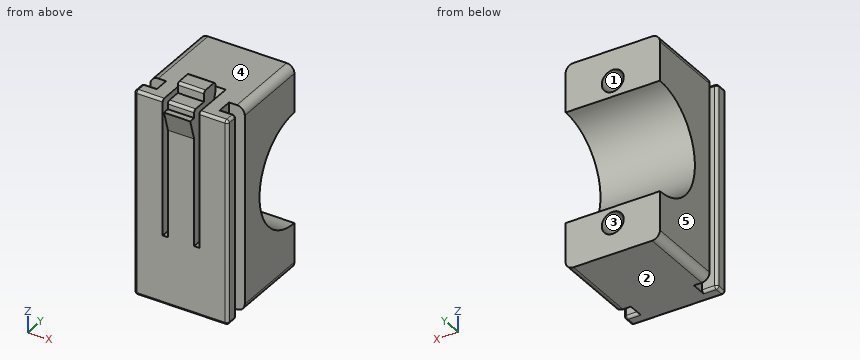
from build123d import *

# Parameters (mm, degrees)
BOSS_EXTRUDE1_DEPTH             = 39
HANDLEBARHOLE_R                 = 10.55
CUT_EXTRUDE1_DEPTH              = 48.381430962
SKETCH3_R                       = 2.1
CUT_EXTRUDE2_DEPTH              = 14
BOSS_EXTRUDE2_DEPTH             = 2.5
BOSS_EXTRUDE2_DEPTH_BACK        = 2.5
FILLET1_R                       = 0.5
CUT_EXTRUDE_THIN2_START         = -3.5
CUT_EXTRUDE_THIN2_DEPTH         = 7
CUT_EXTRUDE5_REACH              = 49.381
SKETCH10_W                      = 1
SKETCH10_H                      = 25.953669743
BOSS_EXTRUDE3_REACH             = 46.744
BOSS_EXTRUDE3_DIRECTION_2_REACH = 46.744
FILLET5_R                       = 1.5


# Read off the part's stored shape, not the designer's step: Cut-Extrude-Thin2
with BuildPart() as part:
    # Sketch1 → Boss-Extrude1 (new body)
    with BuildSketch(Plane.XY):
        Polygon((0, 5), (0, 20), (18, 20), (18, 5), (15, 5), (15, 2.5), (17.9, 2.5), (17.9, 0), (0.1, 0), (0.1, 2.5), (3, 2.5), (3, 5), align=None)
    extrude(amount=BOSS_EXTRUDE1_DEPTH)

    # HandlebarHole → Cut-Extrude1 (cut, through all)
    with BuildSketch(Plane(origin=(0, 0, 0), x_dir=(0, 0, -1), z_dir=(1, 0, 0))):
        with Locations((-19.5, 20)):
            Circle(HANDLEBARHOLE_R)
    extrude(amount=CUT_EXTRUDE1_DEPTH, mode=Mode.SUBTRACT)

    # Sketch3 → Cut-Extrude2 (cut)
    with BuildSketch(Plane(origin=(0, 20, 0), x_dir=(1, 0, 0), z_dir=(0, 1, 0))):
        with Locations(Location((9, -5.95, 0), (0, 0, 270))):
            Circle(SKETCH3_R)
        with Locations(Location((9, -33.05, 0), (0, 0, 270))):
            Circle(SKETCH3_R)
    extrude(amount=-CUT_EXTRUDE2_DEPTH, mode=Mode.SUBTRACT)

    # Sketch4 → Boss-Extrude2 (add, two sides: drawn at the far end of the back side and taken through both)
    with BuildSketch(Plane.ZY.offset(-9).offset(-BOSS_EXTRUDE2_DEPTH_BACK)):
        Polygon((33.5, 0), (37.5, 0), (37.5, -1.2), align=None)
    extrude(amount=BOSS_EXTRUDE2_DEPTH + BOSS_EXTRUDE2_DEPTH_BACK)

    # Fillet1
    fillet1_edges = [part.edges().sort_by_distance(p)[0] for p in [
        (17.9, 1.25, 39),
        (1.55, 2.5, 0),
        (16.45, 2.5, 39),
        (16.45, 2.5, 0),
        (17.9, 1.25, 0),
        (9, 0, 0),
        (0.1, 1.25, 0),
        (0.1, 2.5, 19.5),
        (17.9, 2.5, 19.5),
        (17.9, 0, 19.5),
        (0.1, 0, 19.5),
        (1.55, 2.5, 39),
        (0.1, 1.25, 39),
        (9, 0, 39),
    ]]
    fillet(fillet1_edges, radius=FILLET1_R)

    # Cut-Extrude-Thin2 outline → Cut-Extrude-Thin2 (cut)
    with BuildSketch(Plane.ZY.offset(-9).offset(CUT_EXTRUDE_THIN2_START)):
        with BuildLine():
            add(Edge.make_bspline(
                [(39, 6.377827527), (26.271218228, 2.589898365), (13, 3)],
                knots=[0.07295309, 0.07295309, 0.07295309, 1, 1, 1], degree=2))
            Line((39, 6.377827527), (39.000000003, 7.944068421))
            add(Edge.make_bspline(
                [(39.000000003, 7.944068421), (36.434479895, 7.165477311), (33.853278683, 6.517493693), (31.255701113, 6)],
                knots=[0.057086213, 0.057086213, 0.057086213, 0.057086213, 0.342626571, 0.342626571, 0.342626571, 0.342626571], degree=3))
            add(Edge.make_bspline(
                [(31.255701113, 6), (25.275536046, 4.808621641), (19.208573603, 4.308861265), (13.046330257, 4.499284332)],
                knots=[0.342626571, 0.342626571, 0.342626571, 0.342626571, 1, 1, 1, 1], degree=3))
            Line((13.046330257, 4.499284332), (13, 3))
        make_face()
    extrude(amount=CUT_EXTRUDE_THIN2_DEPTH, mode=Mode.SUBTRACT)

    # Sketch10 → Cut-Extrude5 (cut, up to next)
    with BuildSketch(Plane(origin=(0, 0, 0), x_dir=(1, 0, 0), z_dir=(0, 1, 0)), mode=Mode.PRIVATE) as cut_extrude5_sk1:
        with Locations((12, -26.023165129)):
            Rectangle(SKETCH10_W, SKETCH10_H)
    cut_extrude5_tool1 = extrude(cut_extrude5_sk1.sketch, amount=CUT_EXTRUDE5_REACH, mode=Mode.PRIVATE) & part.part
    # Sketch10 → Cut-Extrude5 (cut, up to next)
    with BuildSketch(Plane(origin=(0, 0, 0), x_dir=(1, 0, 0), z_dir=(0, 1, 0)), mode=Mode.PRIVATE) as cut_extrude5_sk2:
        with Locations((6, -26.023165129)):
            Rectangle(SKETCH10_W, SKETCH10_H)
    cut_extrude5_tool2 = extrude(cut_extrude5_sk2.sketch, amount=CUT_EXTRUDE5_REACH, mode=Mode.PRIVATE) & part.part
    add(cut_extrude5_tool1.solids().sort_by_distance((12, 0, 26.023165))[0], mode=Mode.SUBTRACT)
    add(cut_extrude5_tool2.solids().sort_by_distance((6, 0, 26.023165))[0], mode=Mode.SUBTRACT)

    # Boss-Extrude3: up to this face of the body (flat: up to its plane)
    boss_extrude3_end = Plane(part.part.faces().sort_by_distance((6.5, 2.064317156, 28.033592375))[0])
    # Sketch11 → Boss-Extrude3 (add, up to the picked face)
    with BuildSketch(Plane.ZY.offset(-9), mode=Mode.PRIVATE) as boss_extrude3_sk1:
        with BuildLine():
            Line((39, 3), (40.51, 3))
            ThreePointArc((40.51, 3), (40.856482323, 3.143517677), (41, 3.49))
            Line((41, 3.49), (41, 5.887827527))
            ThreePointArc((41, 5.887827527), (40.856482323, 6.23430985), (40.51, 6.377827527))
            Line((40.51, 6.377827527), (39, 6.377827527))
            Line((39, 6.377827527), (39, 3))
        make_face()
    boss_extrude3_tool1 = split(extrude(boss_extrude3_sk1.sketch, amount=BOSS_EXTRUDE3_REACH, mode=Mode.PRIVATE), bisect_by=boss_extrude3_end, keep=Keep.BOTH, mode=Mode.PRIVATE)
    add(boss_extrude3_tool1.solids().sort_by(Axis((9, 4.688914, 39.986205), (-1, 0, 0)))[0])

    # Boss-Extrude3 direction 2: up to this face of the body (flat: up to its plane)
    boss_extrude3_direction_2_end = Plane(part.part.faces().sort_by_distance((11.5, 2.064317156, 28.033592375))[0])
    # Sketch11 → Boss-Extrude3 direction 2 (add, up to the picked face)
    with BuildSketch(Plane.ZY.offset(-9), mode=Mode.PRIVATE) as boss_extrude3_direction_2_sk1:
        with BuildLine():
            Line((39, 3), (40.51, 3))
            ThreePointArc((40.51, 3), (40.856482323, 3.143517677), (41, 3.49))
            Line((41, 3.49), (41, 5.887827527))
            ThreePointArc((41, 5.887827527), (40.856482323, 6.23430985), (40.51, 6.377827527))
            Line((40.51, 6.377827527), (39, 6.377827527))
            Line((39, 6.377827527), (39, 3))
        make_face()
    boss_extrude3_direction_2_tool1 = split(extrude(boss_extrude3_direction_2_sk1.sketch, amount=-BOSS_EXTRUDE3_DIRECTION_2_REACH, mode=Mode.PRIVATE), bisect_by=boss_extrude3_direction_2_end, keep=Keep.BOTH, mode=Mode.PRIVATE)
    add(boss_extrude3_direction_2_tool1.solids().sort_by(Axis((9, 4.688914, 39.986205), (1, 0, 0)))[0])

    # Fillet5
    fillet5_edges = [part.edges().sort_by_distance(p)[0] for p in [
        (0, 12.5, 0),
        (18, 12.5, 0),
        (18, 12.5, 39),
        (0, 12.5, 39),
    ]]
    fillet(fillet5_edges, radius=FILLET5_R)


solid = part.part
Design review of the part built by this model. Coordinates are the model's own, in mm. Face numbers are marked on the shaded views. A direction names the side the tool comes from. Give positions to 0.01 mm unless a question says otherwise; leave off trailing zeros. Order: outer loops, then holes, each group sorted by start corner. A loop starts at its lowest first (then second) coordinate and runs counter-clockwise, first axis right, second up.
1. Add section D-D, the plane z = 33.05. State how many separate pieces and enclosed holes the cut face has, then the cut area to 3 significant figures.
Solution:
separate pieces: 3
enclosed holes: 0
area: 267 mm2
2. For pin 1 Ø2 at (x, y) = (8, 1.5) entering from +Z; pin 2 Ø2.5 at (y, z) = (1, 33) entering from +X; pin 3 Ø1.9 at (x, z) = (16, 18.5) entering from +Y, all flat-tipped, find the tip position at first contact; note any pin that passes through.
Solution:
pin 1: stops at z = 39
pin 2: stops at x = 17.9
pin 3: stops at y = 9.63
3. Mouldability with a two-part tool opening along X and no side actions: class the marked faces 3, 4 and 5 as +X half, -X half, draft (parallel to the pull), parting line (faces both ways), or undercut.
Solution:
face 3: undercut
face 4: draft
face 5: -X half
4. Tool access review of the marked faces 1 and 2: name each direction out of +Z, -Z, +X, -X, +Y, -Y from which nothing blocks a thin tool from reaching the whole face with its end or side.
Solution:
face 1: +Y
face 2: -Z, +X, -X, +Y, -Y
5. To check wall thickness, follow L1, parallel to X at y = 1.5, z = 15.5; L2, parallel to X at y = 14.5, z = 33.05; L3, parallel to Z at x = 5, y = 7.75. State the ranges of each line that lie inside material, in increasing order.
Solution:
L1: x = 0.1 to 5.5, 6.5 to 11.5, 12.5 to 17.9
L2: x = 0 to 6.9, 11.1 to 18
L3: z = 0 to 39
6. Add section C-C, the plane x = 13.75. State the section outline as (y, z) points.
Solution:
outline: (0, 0.5) arc R0.5 ccw to (0.5, 0) - (20, 0) - (20, 8.95) arc R10.55 cw to (20, 30.05) - (20, 39) - (0.5, 39) arc R0.5 ccw to (0, 38.5) - close
7. Add section B-B, the plane z = 5.95. State the section outline as (x, y) points.
Solution:
outline: (0, 5) - (3, 5) - (3, 2.5) - (0.6, 2.5) arc R0.5 ccw to (0.1, 2) - (0.1, 0.5) arc R0.5 ccw to (0.6, 0) - (17.4, 0) arc R0.5 ccw to (17.9, 0.5) - (17.9, 2) arc R0.5 ccw to (17.4, 2.5) - (15, 2.5) - (15, 5) - (18, 5) - (18, 20) - (11.1, 20) - (11.1, 6) - (6.9, 6) - (6.9, 20) - (0, 20) - close
8. Add section A-A, the plane y = 10.25. State the section outline as (x, z) points, then the cut area to 3 significant figures.
Solution:
outline: (0, 1.5) arc R1.5 ccw to (1.5, 0) - (16.5, 0) arc R1.5 ccw to (18, 1.5) - (18, 15.47) - (0, 15.47) - close; (0, 23.53) - (18, 23.53) - (18, 37.5) arc R1.5 ccw to (16.5, 39) - (1.5, 39) arc R1.5 ccw to (0, 37.5) - close; hole circle Ø4.2 at (9, 5.95); hole circle Ø4.2 at (9, 33.05)
area: 527 mm2
